For this review, take the finished solid that the model builds, in its own axes (mm). A direction names the side the tool comes from. Round coordinates to 2 decimals unless told otherwise and drop trailing zeros. Order: outer loops, then holes, each group sorted by start corner. A loop starts at its lowest first (then second) coordinate and runs counter-clockwise, first axis right, second up. Notation, with made-up numbers: (-23.5, 24.25) - (-12.5, 24.25) arc R6 ccw to (-12.5, 31.25) - close; hole circle Ø9 at (-2, 33). An arc over 180 degrees is marked (long way). One line per question, with ' | ' between items.
```python
from build123d import *

# Parameters (mm, degrees)
BOSS_EXTRU_1_DEPTH      = 15
BOSS_EXTRU_2_START      = -7.5
BOSS_EXTRU_2_DEPTH      = 14.913164891
BOSS_EXTRU_2_START_2    = -7.586835109
BOSS_EXTRU_2_2_DEPTH    = 0.086835109
BOSS_EXTRU_2_START_3    = 7.413164891
BOSS_EXTRU_2_3_DEPTH    = 0.086835109
BOSS_EXTRU_3_DEPTH      = 7.5
BOSS_EXTRU_3_DEPTH_BACK = 7.5
ESQUISSE6_R             = 1.5
ENL_V_MAT_EXTRU_1_DEPTH = 15
ESQUISSE7_R             = 2.5
ENL_V_MAT_EXTRU_2_DEPTH = 7.5
ESQUISSE8_R             = 23.75
ESQUISSE8_R_2           = 14.05
ENL_V_MAT_EXTRU_3_DEPTH = 5.1
ENL_V_MAT_EXTRU_4_DEPTH = 9
ESQUISSE15_W            = 7.790942256
ESQUISSE15_H            = 7.790942256
ESQUISSE15_R            = 3
ENL_V_MAT_EXTRU_5_DEPTH = 2
ENL_V_MAT_EXTRU_6_DEPTH = 5
BOSS_EXTRU_6_START      = 4
ESQUISSE18_R            = 14.05
BOSS_EXTRU_6_DEPTH      = 4


# Read off the part's stored shape, not the designer's step: Boss.-Extru.2
with BuildPart() as part:
    # Esquisse1 → Boss.-Extru.1 (new body)
    with BuildSketch(Plane.XY):
        Polygon((49.913164891, 50), (-50.086835109, 50), (-50.086835109, 0), (-50.086835109, -50), (49.913164891, -50), (49.913164891, 0), align=None)
    extrude(amount=BOSS_EXTRU_1_DEPTH)

    # Boss.-Extru.2 outline → Boss.-Extru.2 (add)
    with BuildSketch(Plane.YZ.offset(BOSS_EXTRU_2_START)):
        Polygon((50, 0), (65, 15), (50, 15), align=None)
        Polygon((-50, 0), (-50, 15), (-65, 15), align=None)
    extrude(amount=BOSS_EXTRU_2_DEPTH)

    # Boss.-Extru.2 2 outline → Boss.-Extru.2 2 (add)
    with BuildSketch(Plane.YZ.offset(BOSS_EXTRU_2_START_2)):
        Polygon((50, 0), (65, 15), (50, 15), align=None)
    extrude(amount=BOSS_EXTRU_2_2_DEPTH)

    # Boss.-Extru.2 3 outline → Boss.-Extru.2 3 (add)
    with BuildSketch(Plane.YZ.offset(BOSS_EXTRU_2_START_3)):
        Polygon((-50, 0), (-50, 15), (-65, 15), align=None)
    extrude(amount=BOSS_EXTRU_2_3_DEPTH)

    # Esquisse4 → Boss.-Extru.3 (add, two sides: drawn at the far end of the back side and taken through both)
    with BuildSketch(Plane(origin=(0, 0, 0), x_dir=(1, 0, 0), z_dir=(0, 1, 0)).offset(-BOSS_EXTRU_3_DEPTH_BACK)):
        Polygon((-50.086835109, 0), (-50.086835109, -15), (-65.086835109, -15), align=None)
        Polygon((49.913164891, 0), (49.913164891, -15), (64.913164891, -15.393130345), align=None)
    extrude(amount=BOSS_EXTRU_3_DEPTH + BOSS_EXTRU_3_DEPTH_BACK)

    # Esquisse6 → Enlèv. mat.-Extru.1 (cut)
    with BuildSketch(Plane(origin=(0, 0, 0), x_dir=(-1, 0, 0), z_dir=(0, 0, -1))):
        with Locations((0, -56)):
            Circle(ESQUISSE6_R)
        with Locations((56.086835109, 0)):
            Circle(ESQUISSE6_R)
        with Locations((0, 56)):
            Circle(ESQUISSE6_R)
        with Locations((-55.913164891, 0)):
            Circle(ESQUISSE6_R)
    extrude(amount=-ENL_V_MAT_EXTRU_1_DEPTH, mode=Mode.SUBTRACT)

    # Esquisse7 → Enlèv. mat.-Extru.2 (cut)
    with BuildSketch(Plane(origin=(0, 0, 0), x_dir=(-1, 0, 0), z_dir=(0, 0, -1))):
        with Locations((56.086835109, 0)):
            Circle(ESQUISSE7_R)
        with Locations((0, 56)):
            Circle(ESQUISSE7_R)
        with Locations((-55.913164891, 0)):
            Circle(ESQUISSE7_R)
        with Locations((0, -56)):
            Circle(ESQUISSE7_R)
    extrude(amount=-ENL_V_MAT_EXTRU_2_DEPTH, mode=Mode.SUBTRACT)

    # Esquisse8 → Enlèv. mat.-Extru.3 (cut)
    with BuildSketch(Plane(origin=(0, 0, 0), x_dir=(-1, 0, 0), z_dir=(0, 0, -1))):
        Circle(ESQUISSE8_R)
        Circle(ESQUISSE8_R_2, mode=Mode.SUBTRACT)
    extrude(amount=-ENL_V_MAT_EXTRU_3_DEPTH, mode=Mode.SUBTRACT)

    # Esquisse11 → Enlèv. mat.-Extru.4 (cut)
    with BuildSketch(Plane(origin=(0, 0, 0), x_dir=(-1, 0, 0), z_dir=(0, 0, -1))):
        Polygon((23.724937024, -1.090808521), (23.708156389, 1.409191479), (31.708156389, 1.462889508), (31.724937024, -1.037110492), align=None)
        Polygon((-31.724937024, -1.037110492), (-31.708156389, 1.462889508), (-23.708156389, 1.409191479), (-23.724937024, -1.090808521), align=None)
    extrude(amount=-ENL_V_MAT_EXTRU_4_DEPTH, mode=Mode.SUBTRACT)

    # Esquisse15 → Enlèv. mat.-Extru.5 (cut)
    # profile 1 of 7: a face of its own
    with BuildSketch(Plane(origin=(0, 0, 0), x_dir=(-1, 0, 0), z_dir=(0, 0, -1))):
        Polygon((0, 5.509028101), (-1.495471128, 3.895471128), (1.495471128, 3.895471128), align=None)
    # profile 2 of 7: a face of its own
    with BuildSketch(Plane(origin=(0, 0, 0), x_dir=(-1, 0, 0), z_dir=(0, 0, -1))):
        Polygon((-3.895471128, -1.495471128), (-3.895471128, 1.495471128), (-5.509028101, 0), align=None)
    # profile 3 of 7: a face of its own
    with BuildSketch(Plane(origin=(0, 0, 0), x_dir=(-1, 0, 0), z_dir=(0, 0, -1))):
        Polygon((1.495471128, -3.895471128), (-1.495471128, -3.895471128), (0, -5.509028101), align=None)
    # profile 4 of 7: a face of its own
    with BuildSketch(Plane(origin=(0, 0, 0), x_dir=(-1, 0, 0), z_dir=(0, 0, -1))):
        Polygon((5.509028101, 0), (3.895471128, 1.495471128), (3.895471128, -1.495471128), align=None)
    # profile 5 of 7: a face of its own
    with BuildSketch(Plane(origin=(0, 0, 0), x_dir=(-1, 0, 0), z_dir=(0, 0, -1))):
        Rectangle(ESQUISSE15_W, ESQUISSE15_H)
        Circle(ESQUISSE15_R, mode=Mode.SUBTRACT)
    # profile 6 of 7: a face of its own
    with BuildSketch(Plane(origin=(0, 0, 0), x_dir=(-1, 0, 0), z_dir=(0, 0, -1))):
        with BuildLine():
            ThreePointArc((3, 0), (0.776457135, 2.897777479), (-2.598076211, 1.5))
            Line((-2.598076211, 1.5), (-2.598076211, -1.5))
            ThreePointArc((-2.598076211, -1.5), (0.776457135, -2.897777479), (3, 0))
        make_face()
    # profile 7 of 7: a face of its own
    with BuildSketch(Plane(origin=(0, 0, 0), x_dir=(-1, 0, 0), z_dir=(0, 0, -1))):
        with BuildLine():
            Line((-2.598076211, -1.5), (-2.598076211, 1.5))
            ThreePointArc((-2.598076211, 1.5), (-3, 0), (-2.598076211, -1.5))
        make_face()
    extrude(amount=-ENL_V_MAT_EXTRU_5_DEPTH, mode=Mode.SUBTRACT)

    # Esquisse17 → Enlèv. mat.-Extru.6 (cut)
    with BuildSketch(Plane(origin=(0, 0, 2), x_dir=(-1, 0, 0), z_dir=(0, 0, -1))):
        with BuildLine():
            ThreePointArc((3.15, 0), (1.220286151, 2.904031975), (-2.204540769, 2.25))
            Line((-2.204540769, 2.25), (-2.204540769, -2.25))
            ThreePointArc((-2.204540769, -2.25), (1.220286151, -2.904031975), (3.15, 0))
        make_face()
    extrude(amount=-ENL_V_MAT_EXTRU_6_DEPTH, mode=Mode.SUBTRACT)

    # Esquisse18 → Boss.-Extru.6 (add)
    with BuildSketch(Plane(origin=(0, 0, 0), x_dir=(-1, 0, 0), z_dir=(0, 0, -1)).offset(BOSS_EXTRU_6_START)):
        Circle(ESQUISSE18_R)
        Polygon((0, 5.509028101), (1.495471128, 3.895471128), (3.895471128, 3.895471128), (3.895471128, 1.495471128), (5.509028101, 0), (3.895471128, -1.495471128), (3.895471128, -3.895471128), (1.495471128, -3.895471128), (0, -5.509028101), (-1.495471128, -3.895471128), (-3.895471128, -3.895471128), (-3.895471128, -1.495471128), (-5.509028101, 0), (-3.895471128, 1.495471128), (-3.895471128, 3.895471128), (-1.495471128, 3.895471128), align=None, mode=Mode.SUBTRACT)
    extrude(amount=-BOSS_EXTRU_6_DEPTH)


solid = part.part
```
(1) We need section B-B on y = -19. State the section outline as (x, z) points, plus the area to 3 significant figures.
Output values:
outline: (-50.09, 0) - (-14.25, 0) - (-14.25, 5.1) - (14.25, 5.1) - (14.25, 0) - (49.91, 0) - (49.91, 15) - (-50.09, 15) - close | area: 1,350 mm^2
(2) We need section A-A on y = 56. State the section outline as (x, z) points, plus the area to 3 significant figures.
Output values:
outline: (-7.59, 6) - (-2.5, 6) - (-2.5, 7.5) - (-1.5, 7.5) - (-1.5, 15) - (-7.59, 15) - close; (1.5, 7.5) - (2.5, 7.5) - (2.5, 6) - (7.41, 6) - (7.41, 15) - (1.5, 15) - close | area: 105 mm^2
(3) For faces 1 (the flat face through (29, 50, 7)), 2 (the flat face through (-7.587, 56, 9)), 3 (the flat face through (7.5, -54, 11)), list the 3-axis set-ups (+Z, -Z, +X, -X, +Y, -Y) from which the entire face can be reached by the end or side of a thin tool; tool diameter is ignored.
Output values:
face 1: +Z, -Z, +X, +Y | face 2: +Z, -Z, -X, +Y | face 3: +Z, -Z, +X, -Y
(4) Insertion check: pin 1 (3 mm diameter, centred on y = -17, z = 2.5, fed in from -X); pin 2 (8 mm diameter, centred on x = -8.5, y = -4, fed in from +Z); pin 3 (6 mm diameter, centred on x = 0, y = -56, fed in from -Z); pin 4 (1.8 mm diameter, centred on x = 0, y = -56, fed in from +Z). Each pin has a flat end and moves straight along its axis. Give the tip position at first contact, or say it passes through.
Output values:
pin 1: x = -50.09 | pin 2: z = 15 | pin 3: z = 3 | pin 4: through
(5) We need section D-D on y = 40.5. State the section outline as (x, z) points, plus the area to 3 significant figures.
Output values:
outline: (-50.09, 0) - (49.91, 0) - (49.91, 15) - (-50.09, 15) - close | area: 1,500 mm^2
(6) We need section C-C on x = -20. State the section outline as (y, z) points, plus the area to 3 significant figures.
Output values:
outline: (-50, 0) - (-12.81, 0) - (-12.81, 5.1) - (12.81, 5.1) - (12.81, 0) - (50, 0) - (50, 15) - (-50, 15) - close | area: 1,370 mm^2
(7) For probe 1 along Y at (x, z) = (0, 4.55); probe 2 along Y at (x, z) = (0, 11.5); probe 3 along Y at (x, z) = (0, 5.8), list the stretches that pass through material, from the lowest coordinate up. Write a range as [from, to].
Output values:
probe 1: [-53.5, -23.75], [-14.05, -3.15], [3.15, 14.05], [23.75, 53.5] | probe 2: [-61.5, -57.5], [-54.5, 54.5], [57.5, 61.5] | probe 3: [-53.5, -3.15], [3.15, 53.5]
